Geometry: final body of the model. Coordinates: model frame, mm. A direction names the side the tool comes from. Round coordinates to 2 decimals unless told otherwise and drop trailing zeros. Loops run counter-clockwise (first coordinate to the right, second up) from the corner with the lowest first, then second, coordinate; pieces in that order, holes last. Notation, with made-up numbers: M 23.25,70.5 L 48.25,70.5 A9 ccw 48.25,76.5 Z; hole C 45,74.5 d8. An arc over 180 degrees is marked long. Return JSON: item names as keys, results as strings.
from build123d import *

# Parameters (mm, degrees)
BOSS_EXTRUDE1_DEPTH     = 12.5
SKETCH2_W               = 10.7
SKETCH2_H               = 41.65
BOSS_EXTRUDE2_DEPTH     = 5
CUT_EXTRUDE1_DEPTH      = 19.7
CUT_EXTRUDE1_DEPTH_BACK = 6
CUT_EXTRUDE2_START      = 4
CUT_EXTRUDE2_DEPTH      = 3


with BuildPart() as part:
    # Sketch1 → Boss-Extrude1 (new body, symmetric)
    with BuildSketch(Plane(origin=(0, 0, 0), x_dir=(0, 0, -1), z_dir=(1, 0, 0))):
        with BuildLine():
            Line((0, 0), (70, 0))
            Line((70, 0), (70, 8.7))
            ThreePointArc((70, 8.7), (60, 18.7), (50, 8.7))
            Line((50, 8.7), (50, 4))
            Line((50, 4), (20, 4))
            Line((20, 4), (20, 8.7))
            ThreePointArc((20, 8.7), (10, 18.7), (0, 8.7))
            Line((0, 8.7), (0, 0))
        make_face()
    extrude(amount=BOSS_EXTRUDE1_DEPTH, both=True)

    # Sketch2 → Boss-Extrude2 (add)
    with BuildSketch(Plane(origin=(0, 0, 0), x_dir=(1, 0, 0), z_dir=(0, 1, 0))):
        with BuildLine():
            ThreePointArc((-5.35, 41.65), (0, 47), (5.35, 41.65))
            Line((5.35, 41.65), (-5.35, 41.65))
        make_face()
        with Locations((0, 20.825)):
            Rectangle(SKETCH2_W, SKETCH2_H)
    extrude(amount=-BOSS_EXTRUDE2_DEPTH)

    # Sketch4 → Cut-Extrude1 (cut, two sides)
    with BuildSketch(Plane(origin=(0, 0, 0), x_dir=(1, 0, 0), z_dir=(0, 1, 0))) as cut_extrude1_sk:
        with BuildLine():
            Line((-1.625, 40), (1.625, 40))
            Line((1.625, 40), (1.625, 46))
            ThreePointArc((1.625, 46), (0, 47.625), (-1.625, 46))
            Line((-1.625, 46), (-1.625, 40))
        make_face()
        with BuildLine():
            Line((1.625, 38.100164481), (1.625, 40))
            ThreePointArc((1.625, 40), (0, 38.375), (-1.625, 40))
            Line((-1.625, 40), (-1.625, 38.100164481))
            ThreePointArc((-1.625, 38.100164481), (0, 37.5), (1.625, 38.100164481))
        make_face()
        with BuildLine():
            ThreePointArc((-1.625, 40), (0, 38.375), (1.625, 40))
            Line((1.625, 40), (-1.625, 40))
        make_face()
        with BuildLine():
            Line((1.625, 32.899835519), (1.625, 38.100164481))
            ThreePointArc((1.625, 38.100164481), (0, 37.5), (-1.625, 38.100164481))
            Line((-1.625, 38.100164481), (-1.625, 32.899835519))
            ThreePointArc((-1.625, 32.899835519), (0, 33.5), (1.625, 32.899835519))
        make_face()
        with BuildLine():
            ThreePointArc((-1.625, 31), (0, 32.625), (1.625, 31))
            Line((1.625, 31), (1.625, 32.899835519))
            ThreePointArc((1.625, 32.899835519), (0, 33.5), (-1.625, 32.899835519))
            Line((-1.625, 32.899835519), (-1.625, 31))
        make_face()
        with BuildLine():
            Line((-1.625, 31), (1.625, 31))
            ThreePointArc((1.625, 31), (0, 32.625), (-1.625, 31))
        make_face()
        with BuildLine():
            Line((1.625, 25), (1.625, 31))
            Line((1.625, 31), (-1.625, 31))
            Line((-1.625, 31), (-1.625, 25))
            ThreePointArc((-1.625, 25), (0, 23.375), (1.625, 25))
        make_face()
    extrude(amount=CUT_EXTRUDE1_DEPTH, mode=Mode.SUBTRACT)
    extrude(cut_extrude1_sk.sketch, amount=-CUT_EXTRUDE1_DEPTH_BACK, mode=Mode.SUBTRACT)

    # Sketch4<3> → Cut-Extrude2 (cut)
    with BuildSketch(Plane(origin=(0, 0, 0), x_dir=(1, 0, 0), z_dir=(0, 1, 0)).offset(CUT_EXTRUDE2_START)):
        with BuildLine():
            Line((2.5, 25), (2.5, 31))
            Line((2.5, 31), (1.625, 31))
            Line((1.625, 31), (1.625, 25))
            ThreePointArc((1.625, 25), (0, 23.375), (-1.625, 25))
            Line((-1.625, 25), (-1.625, 31))
            Line((-1.625, 31), (-2.5, 31))
            Line((-2.5, 31), (-2.5, 25))
            ThreePointArc((-2.5, 25), (0, 22.5), (2.5, 25))
        make_face()
        with BuildLine():
            ThreePointArc((-1.625, 32.899835519), (-2.270737766, 32.045825033), (-2.5, 31))
            Line((-2.5, 31), (-1.625, 31))
            Line((-1.625, 31), (-1.625, 32.899835519))
        make_face()
        with BuildLine():
            ThreePointArc((-1.625, 38.100164481), (-2.270737766, 38.954174967), (-2.5, 40))
            Line((-2.5, 40), (-2.5, 31))
            ThreePointArc((-2.5, 31), (-2.270737766, 32.045825033), (-1.625, 32.899835519))
            Line((-1.625, 32.899835519), (-1.625, 38.100164481))
        make_face()
        with BuildLine():
            Line((1.625, 31), (2.5, 31))
            ThreePointArc((2.5, 31), (2.270737766, 32.045825033), (1.625, 32.899835519))
            Line((1.625, 32.899835519), (1.625, 31))
        make_face()
        with BuildLine():
            Line((2.5, 31), (2.5, 40))
            ThreePointArc((2.5, 40), (2.270737766, 38.954174967), (1.625, 38.100164481))
            Line((1.625, 38.100164481), (1.625, 32.899835519))
            ThreePointArc((1.625, 32.899835519), (2.270737766, 32.045825033), (2.5, 31))
        make_face()
        with BuildLine():
            ThreePointArc((1.625, 38.100164481), (2.270737766, 38.954174967), (2.5, 40))
            Line((2.5, 40), (1.625, 40))
            Line((1.625, 40), (1.625, 38.100164481))
        make_face()
        with BuildLine():
            Line((2.5, 40), (2.5, 46))
            ThreePointArc((2.5, 46), (0, 48.5), (-2.5, 46))
            Line((-2.5, 46), (-2.5, 40))
            Line((-2.5, 40), (-1.625, 40))
            Line((-1.625, 40), (-1.625, 46))
            ThreePointArc((-1.625, 46), (0, 47.625), (1.625, 46))
            Line((1.625, 46), (1.625, 40))
            Line((1.625, 40), (2.5, 40))
        make_face()
        with BuildLine():
            Line((-1.625, 40), (-2.5, 40))
            ThreePointArc((-2.5, 40), (-2.270737766, 38.954174967), (-1.625, 38.100164481))
            Line((-1.625, 38.100164481), (-1.625, 40))
        make_face()
    extrude(amount=-CUT_EXTRUDE2_DEPTH, mode=Mode.SUBTRACT)


solid = part.part
Q1. Section query C-C (x = 0). Output: boundary loops of the cut face in (y, z) (3 decimals).
Determined:
{"outline": "M -5,-23.375 L 1,-23.375 L 1,-22.5 L 4,-22.5 L 4,-20 L 8.7,-20 A10 ccw 8.7,0 L -5,0 Z; M 0,-70 L 8.7,-70 A10 ccw 8.7,-50 L 4,-50 L 4,-48.5 L 1,-48.5 L 1,-47.625 L 0,-47.625 Z"}
Q2. Material intervals for L1, parallel to Z at x = -9.25, y = 9; L2, parallel to X at y = 3, z = -45; L3, parallel to Z at x = -7, y = 16.5, sorted ascending.
Determined:
{"L1": "z = -70 to -50, -20 to 0", "L2": "x = -12.5 to -2.5, 2.5 to 12.5", "L3": "z = -66.26 to -53.74, -16.26 to -3.74"}
Q3. Section query B-B (z = -35.5). Output: boundary loops of the cut face in (x, y) (3 decimals).
Determined:
{"outline": "M -12.5,0 L -5.35,0 L -5.35,-5 L -1.625,-5 L -1.625,1 L -2.5,1 L -2.5,4 L -12.5,4 Z; M 1.625,-5 L 5.35,-5 L 5.35,0 L 12.5,0 L 12.5,4 L 2.5,4 L 2.5,1 L 1.625,1 Z"}
Q4. Pull-direction query (Z, two-part tool) for faces 1 (the cylindrical face through (0.2, 18.7, -10.2)), 2 (the cylindrical face through (-4.28, -2.46, -44.86)), 3 (the flat face through (-5.35, -2, -21)); classes: pulls with the +Z half, pulls with the -Z half, needs draft (parallel to the pull), parting line crosses it, or undercut.
Determined:
{"face 1": "undercut", "face 2": "pulls with the -Z half", "face 3": "needs draft"}
Q5. Reachability of faces 4 (the flat face through (-1.625, -2, -36)), 5 (the flat face through (0, 6, -20)), 6 (the flat face through (6, 0, -35)), 7 (the flat face through (5.35, -2, -21)) from +Z, -Z, +X, -X, +Y, -Y: full face, straight path, thin tool, end or side. Return the list, or none.
Determined:
{"face 4": "+Y, -Y", "face 5": "+X, -X, +Y", "face 6": "-Z, -Y", "face 7": "+Z, -Z, +X, -Y"}
Q6. Section query D-D (x = -6.25). Output: boundary loops of the cut face in (y, z), plus the area to 3 significant figures.
Determined:
{"outline": "M 0,-70 L 8.7,-70 A10 ccw 8.7,-50 L 4,-50 L 4,-20 L 8.7,-20 A10 ccw 8.7,0 L 0,0 Z", "area": "782 mm^2"}
Q7. Pin query (flat end, axial travel): pin 1 (2.5 mm diameter, centred on x = -1, z = -40, fed in from +Y); pin 2 (3 mm diameter, centred on y = -2.5, z = -40, fed in from +X); pin 3 (5.5 mm diameter, centred on y = -3, z = -31, fed in from -X). Return the tip coordinate at first contact, or that it passes through.
Determined:
{"pin 1": "stops at y = 1", "pin 2": "stops at x = 5.35", "pin 3": "stops at x = -5.35"}
Q8. Section query A-A (y = 5.25). Output: boundary loops of the cut face in (x, z).
Determined:
{"outline": "M -12.5,-70 L 12.5,-70 L 12.5,-50 L -12.5,-50 Z; M -12.5,-20 L 12.5,-20 L 12.5,0 L -12.5,0 Z"}
